The model under review builds one solid part; all positions refer to its coordinate system, in mm. Face numbers are marked on the shaded views. Coordinates: 2 decimals unless noted, no trailing zeros. Loops run counter-clockwise (first coordinate to the right, second up) from the corner with the lowest first, then second, coordinate; pieces in that order, holes last. Notation, with made-up numbers: (-8, -21) - (10, -21) arc R25 ccw to (10, 8) - close; hole circle Ø7 at (48, 13.25). An arc over 180 degrees is marked (long way). Answer in a Markdown table with one row per item. Add a question column.
(1) For line 1 along Y through (x, z) = (19.5, 3.2); line 2 along Z through (x, y) = (-35, 111); line 3 along Y through (x, z) = (-20, -2), list the stretches that pass through material, from the lowest coordinate up.
(2) We need section B-B on y = 113. Write out the cut boundary in (x, z).
(3) Mouldability with a two-part tool opening along X and no side actions: class the marked faces 1 and 2 as +X half, -X half, draft (parallel to the pull), parting line (faces both ways), or undercut.
(4) For P1, Ø1.5, axis at x = -30, y = 131, coming from the +Z side; P2, Ø4, axis at x = -10.5, z = 2, coming from the -Y side; P3, Ø1.5, axis at x = 32, z = -1, coming from the -Y side; P4, Ø1, axis at x = 2, y = 61.5, coming from the -Z side, all flat-tipped, find the tip position at first contact; note any pin that passes through.
(5) We need section A-A on x = -15.5. Write out the cut boundary in (y, z), plus the area to 3 significant figures.
(6) We need section C-C on y = 15.5. Give the number of separate pieces and of enclosed holes in the cut face, plus the area to 3 significant figures.
Autodesk Inventor part; units mm, degrees
ref_plane "YZ Plane" through (0, 0, 0) normal (1, 0, 0) x (0, 1, 0)
ref_plane "XZ Plane" through (0, 0, 0) normal (0, 1, 0) x (-1, 0, 0)
ref_plane "XY Plane" through (0, 0, 0) normal (0, 0, 1) x (1, 0, 0)
sketch "Sketch1" plane through (0, 0, 0) normal (0, 0, 1) x (1, 0, 0)
  line L0 (-21.25, 21.25) -> (21.25, 21.25)
  line L1 (21.25, 21.25) -> (21.25, -21.25)
  line L2 (21.25, -21.25) -> (-21.25, -21.25)
  line L3 (-21.25, -21.25) -> (-21.25, 21.25)
  line L4 (-21.25, 21.25) -> (21.25, -21.25) construction
  line L5 (21.25, 21.25) -> (-21.25, -21.25) construction
  circle A0 centre (0, 0) radius 11 construction
  circle A1 centre (0, 0) radius 12.5
  line L6 (-25.25, 3.5236) -> (25.25, 3.5236)
  line L7 (25.25, 3.5236) -> (25.25, 25.25)
  line L8 (25.25, 25.25) -> (-25.25, 25.25)
  line L9 (-25.25, 25.25) -> (-25.25, 3.5236)
  circle A2 centre (-15.5, 15.5) radius 1.5
  circle A3 centre (15.5, 15.5) radius 1.5
  point P0 (21.25, 3.5236)
  point P1 (-21.25, 3.5236)
  dimension "d0" = 42.5
  dimension "d1" = 42.5
  dimension "d2" = 22
  dimension "d3" = 25
  dimension "d4" = 4
  dimension "d5" = 4
  dimension "d6" = 4
  dimension "d7" = 3
  dimension "d8" = 3
  dimension "d9" = 15.5
  dimension "d10" = 15.5
  dimension "d11" = 15.5
  dimension "d12" = 15.5
extrude "Extrusion1" add sketch "Sketch1" along normal blind 4 contours L3 L6 L9 L8 L7 L1 L0 | L0 L1 L6 A1 L3 | A1 L6 picked at (3.04, 5.1985)
extrude "Extrusion3" add sketch "Sketch1" against normal blind 8 contours L3 L6 L9 L8 L7 L1 L0
sketch "Sketch2" plane through (0, 0, 4) normal (0, 0, 1) x (1, 0, 0)
  circle A0 centre (0, 0) radius 40 construction
  line L0 (-25.25, 3.5236) -> (25.25, 3.5236) construction
  line L1 (-25.25, 3.5236) -> (25.25, 3.5236)
  line L2 (-25.25, 3.5236) -> (25.25, 3.5236)
  line L3 (39.8445, 92.8978) -> (39.8445, 152.8119)
  line L4 (39.8445, 152.8119) -> (-39.8445, 152.8119)
  line L5 (-39.8445, 152.8119) -> (-39.8445, 82.8978)
  circle A1 centre (-15.5, 15.5) radius 1.5
  circle A2 centre (-15.5, 15.5) radius 1.5
  circle A3 centre (15.5, 15.5) radius 1.5
  circle A4 centre (15.5, 15.5) radius 1.5
  line L6 (25.25, 43.5236) -> (25.25, 3.5236)
  line L7 (25.25, 43.5236) -> (25.25, -31.0232) construction
  line L8 (-25.25, 25.25) -> (-25.25, -31.0232) construction
  line L9 (25.25, 3.5236) -> (25.25, 43.5236)
  line L10 (25.25, 3.5236) -> (25.25, 43.5236) construction
  line L11 (25.25, 43.5236) -> (39.8445, 43.5236) construction
  line L12 (39.8445, 43.5236) -> (39.8445, 92.8978) construction
  spline S0 degree 3 poles (25.25, 3.5236) (25.25, 43.5236) (39.8445, 43.5236) (39.8445, 92.8978) knots 1 1 1 1 2 2 2 2
  line L13 (-25.25, 3.5236) -> (-25.25, 43.5236) construction
  line L14 (-25.25, 43.5236) -> (-39.8445, 43.5236) construction
  line L15 (-39.8445, 43.5236) -> (-39.8445, 82.8978) construction
  spline S1 degree 3 poles (-25.25, 3.5236) (-25.25, 43.5236) (-39.8445, 43.5236) (-39.8445, 82.8978) knots 1 1 1 1 2 2 2 2
  line L16 (34.8445, 168.0706) -> (34.8445, -11.808) construction
  line L17 (-34.8445, 167.0543) -> (-34.8445, -11.808) construction
  line L18 (-29.8445, 168.6418) -> (-29.8445, -10.2205) construction
  line L19 (29.8445, 168.8008) -> (29.8445, -11.0778) construction
  line L20 (41.0033, 130.8119) -> (-56.4356, 130.8119) construction
  circle A5 centre (-29.8445, 130.8119) radius 1.25
  circle A6 centre (29.8445, 130.8119) radius 1.25
  point P0 (-11.9931, 3.5236)
  point P1 (-39.8445, 3.5236)
  point P2 (39.8445, 3.5236)
  dimension "d19" = 80
  dimension "d20" = 150
  dimension "d21" = 39.8445
  dimension "d33" = 40
  dimension "d34" = 40
  dimension "d35" = 40
  dimension "d36" = 39.8445
  dimension "d37" = 5
  dimension "d38" = 5
  dimension "d61" = 10
  dimension "d62" = 10
  dimension "d63" = 22
  dimension "d64" = 2.5
  dimension "d65" = 2.5
extrude "Extrusion4" add sketch "Sketch2" against normal blind 4 contours S1 L5 L4 L3 S0 L1 | A5 | A6
fillet "Fillet1" radius 20 2 edges at (-39.8445, 152.8119, 2) (39.8445, 152.8119, 2)
sketch "Sketch3" plane through (0, 0, 0) normal (0, 0, -1) x (-1, 0, 0)
  line L0 (-40.0079, 28.25) -> (78.3012, 28.25) construction
  line L1 (25.25, 25.25) -> (-25.25, 25.25)
  line L2 (-19.5, 51.7245) -> (-19.5, -25.7194) construction
  line L3 (19.5, 50.7243) -> (19.5, -26.4338) construction
  circle A0 centre (-19.5, 28.25) radius 1.25
  circle A1 centre (19.5, 28.25) radius 1.25
  point P0 (0, 0)
  dimension "d26" = 3
  dimension "d27" = 19.5
  dimension "d28" = 19.5
  dimension "d29" = 2.5
  dimension "d30" = 2.5
extrude "Extrusion5" cut sketch "Sketch3" against normal blind 10
sketch "Sketch4" plane through (0, 0, 0) normal (0, 0, -1) x (-1, 0, 0)
  line L0 (-34.8445, 174.3908) -> (-34.8445, -4.6748) construction
  line L1 (34.8445, 172.891) -> (34.8445, -6.1746) construction
  line L2 (39.8445, 174.885) -> (39.8445, -4.1806) construction
  line L3 (39.8445, 82.8978) -> (39.8445, 132.8119)
  line L4 (-39.8445, 132.8119) -> (-39.8445, 92.8978)
  line L5 (-58.077, 152.8119) -> (62.4518, 152.8119) construction
  line L6 (19.8445, 152.8119) -> (-19.8445, 152.8119)
  line L7 (-60.7578, 80.8119) -> (59.771, 80.8119) construction
  line L8 (-61.2028, 66.8119) -> (59.326, 66.8119) construction
  circle A0 centre (-34.8445, 80.8119) radius 1
  circle A1 centre (-34.8445, 66.8119) radius 1
  circle A2 centre (34.8445, 80.8119) radius 1
  circle A3 centre (34.8445, 66.8119) radius 1
  line L9 (-29.8445, 176.1827) -> (-29.8445, -2.8829) construction
  line L10 (29.8445, 178.0117) -> (29.8445, -1.0539) construction
  line L11 (-58.5074, 88.8119) -> (62.0214, 88.8119) construction
  line L12 (-58.4589, 58.8119) -> (62.0699, 58.8119) construction
  line L13 (-39.8445, 88.8119) -> (-29.8445, 88.8119) construction
  line L14 (-29.8445, 88.8119) -> (-29.8445, 58.8119) construction
  line L15 (-29.8445, 58.8119) -> (-36.5289, 58.8119) construction
  line L16 (-36.5289, 58.7119) -> (-29.7445, 58.7119)
  line L17 (-29.7445, 58.7119) -> (-29.7445, 88.9119)
  line L18 (-29.7445, 88.9119) -> (-39.7987, 88.9119)
  line L19 (-39.8276, 90.9119) -> (-27.7445, 90.9119)
  line L20 (-27.7445, 90.9119) -> (-27.7445, 56.7119)
  line L21 (-27.7445, 56.7119) -> (-36.0331, 56.7119)
  line L22 (-36.5289, 58.7119) -> (-36.0331, 56.7119)
  line L23 (-39.8445, 176.1815) -> (-39.8445, 90.9119) construction
  line L24 (-39.8445, 88.9119) -> (-39.8445, -2.8841) construction
  line L25 (-39.8276, 90.9119) -> (-39.7987, 88.9119)
  line L26 (0, 0) -> (0, 162.0516)
  circle A4 centre (34.8445, 80.8119) radius 1
  circle A5 centre (34.8445, 66.8119) radius 1
  line L27 (39.8445, 88.8119) -> (29.8445, 88.8119) construction
  line L28 (29.8445, 88.8119) -> (29.8445, 58.8119) construction
  line L29 (29.8445, 58.8119) -> (36.5289, 58.8119) construction
  line L30 (36.5289, 58.7119) -> (29.7445, 58.7119)
  line L31 (29.7445, 58.7119) -> (29.7445, 88.9119)
  line L32 (29.7445, 88.9119) -> (39.7987, 88.9119)
  line L33 (39.8276, 90.9119) -> (27.7445, 90.9119)
  line L34 (27.7445, 90.9119) -> (27.7445, 56.7119)
  line L35 (27.7445, 56.7119) -> (36.0331, 56.7119)
  line L36 (36.5289, 58.7119) -> (36.0331, 56.7119)
  line L37 (39.8276, 90.9119) -> (39.7987, 88.9119)
  point P0 (-29.8445, 82.3994)
  point P1 (-29.8445, 68.3994)
  point P2 (29.8445, 83.9869)
  point P3 (29.8445, 69.9869)
  point P4 (-33.257, 88.8119)
  point P5 (36.432, 88.8119)
  point P6 (-33.257, 58.8119)
  point P7 (36.432, 58.8119)
  point P8 (39.8445, 92.8978)
  point P9 (29.8445, 82.3994)
  point P10 (29.8445, 68.3994)
  point P11 (33.257, 88.8119)
  point P12 (33.257, 58.8119)
  point P13 (39.8445, 88.9119)
  point P14 (39.8445, 90.9119)
  dimension "d40" = 5
  dimension "d41" = 72
  dimension "d42" = 14
  dimension "d43" = 2
  dimension "d44" = 2
  dimension "d45" = 2
  dimension "d46" = 2
  dimension "d49" = 5
  dimension "d50" = 5
  dimension "d51" = 8
  dimension "d52" = 8
  dimension "d53" = 0.1
  dimension "d54" = 2
extrude "Extrusion6" cut sketch "Sketch4" against normal blind 10 contours A0 | A1 | A2 | A3
extrude "Extrusion7" add sketch "Sketch4" along normal blind 3 contours L16 L17 L18 L25 L19 L20 L21 L22
extrude "Extrusion8" add sketch "Sketch4" along normal blind 3 contours L36 L35 L34 L33 L37 L32 L31 L30
extrude "Extrusion9" cut sketch "Sketch1" along normal blind 10 contours L6 A1 | A1 L6
extrude "Extrusion10" cut sketch "Sketch2" against normal blind 10 contours A5 | A6
fillet "Fillet3" radius 1 5 edges at (0, 152.8119, 4) (39.8445, 112.8548, 4) (32.5473, 44.6953, 4) (-32.5473, 43.4453, 4) (-39.8445, 107.8548, 4)
sketch "Sketch5" plane through (0, 0, 0) normal (0, 0, -1) x (-1, 0, 0)
  line L0 (4.2555, 165.0839) -> (4.2555, -21.0634) construction
  line L1 (-39.8445, 132.8119) -> (-39.8445, 92.8978) construction
  line L2 (-55.7107, 123.8119) -> (58.0035, 123.8119) construction
  line L3 (-52.844, 69.8119) -> (64.1192, 69.8119) construction
  line L4 (19.8445, 152.8119) -> (-19.8445, 152.8119) construction
  circle A0 centre (4.2555, 123.8119) radius 1.25
  circle A1 centre (4.2555, 69.8119) radius 1.25
  point P0 (0, 0)
  dimension "d69" = 44.1
  dimension "d70" = 29
  dimension "d71" = 83
  dimension "d72" = 2.5
  dimension "d73" = 2.5
extrude "Extrusion11" cut sketch "Sketch5" against normal blind 10
sketch "Sketch6" plane through (0, 0, 4) normal (0, 0, 1) x (1, 0, 0)
  circle A0 centre (-15.5, 15.5) radius 1.5
  circle A1 centre (-15.5, 15.5) radius 3
  circle A2 centre (15.5, 15.5) radius 1.5
  circle A3 centre (15.5, 15.5) radius 3
  circle A4 centre (-29.8445, 130.8119) radius 1.25
  circle A5 centre (-29.8445, 130.8119) radius 2.5
  circle A6 centre (-4.2555, 123.8119) radius 1.25
  circle A7 centre (-4.2555, 123.8119) radius 2.5
  circle A8 centre (29.8445, 130.8119) radius 1.25
  circle A9 centre (29.8445, 130.8119) radius 2.5
  circle A10 centre (-4.2555, 69.8119) radius 1.25
  circle A11 centre (-4.2555, 69.8119) radius 2.5
  circle A12 centre (-19.5, 28.25) radius 1.25
  circle A13 centre (-19.5, 28.25) radius 2.5
  circle A14 centre (19.5, 28.25) radius 1.25
  circle A15 centre (19.5, 28.25) radius 2.5
  circle A16 centre (-34.8445, 80.8119) radius 1
  circle A17 centre (-34.8445, 80.8119) radius 2.25
  circle A18 centre (-34.8445, 66.8119) radius 1
  circle A19 centre (-34.8445, 66.8119) radius 2.25
  circle A20 centre (34.8445, 80.8119) radius 1
  circle A21 centre (34.8445, 80.8119) radius 2.25
  circle A22 centre (34.8445, 66.8119) radius 1
  circle A23 centre (34.8445, 66.8119) radius 2.25
  point P0 (0, 0)
  dimension "d76" = 6
  dimension "d77" = 6
  dimension "d78" = 5
  dimension "d79" = 5
  dimension "d81" = 5
  dimension "d82" = 5
  dimension "d83" = 5
  dimension "d84" = 5
  dimension "d85" = 4.5
  dimension "d86" = 4.5
  dimension "d87" = 4.5
  dimension "d88" = 4.5
extrude "Extrusion12" cut sketch "Sketch6" against normal blind 1
equation "\"d1\" = d0"
equation "\"d5\" = d4"
equation "\"d6\" = d4"
equation "\"d8\" = d7"
equation "\"d11\" = d9"
equation "\"d21\" = d36"
equation "\"d34\" = d33"
equation "\"d35\" = d33"
equation "\"d38\" = d37"
properties part number "Sideplate"
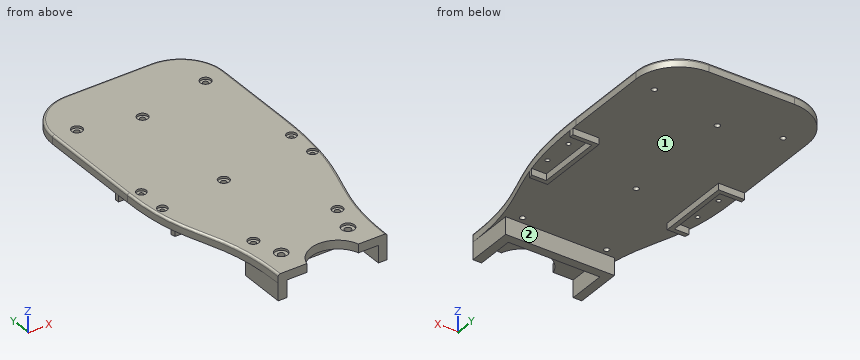
Outcome:
| question | item | result |
|---|---|---|
| 1 | line 1 | 3.52 to 25.75, 30.75 to 152.79 |
| 1 | line 2 | 0 to 4 |
| 1 | line 3 | 21.25 to 25.25 |
| 2 | outline | (-39.84, 0) - (39.84, 0) - (39.84, 3) arc R1 ccw to (38.84, 4) - (-38.84, 4) arc R1 ccw to (-39.84, 3) - close |
| 3 | face 1 | undercut |
| 3 | face 2 | draft |
| 4 | P1 | through |
| 4 | P2 | y = 3.52 |
| 4 | P3 | y = 56.71 |
| 4 | P4 | z = 0 |
| 5 | outline | (3.52, 0) - (14, 0) - (14, 3) - (12.5, 3) - (12.5, 4) - (3.52, 4) - close; (17, 0) - (21.25, 0) - (21.25, -8) - (25.25, -8) - (25.25, 0) - (152.81, 0) - (152.81, 3) arc R1 ccw to (151.81, 4) - (18.5, 4) - (18.5, 3) - (17, 3) - close |
| 5 | area | 614 mm² |
| 6 | separate pieces | 3 |
| 6 | enclosed holes | 0 |
| 6 | area | 240 mm² |
